from build123d import *

# Parameters (mm, degrees)
AUFSATZ_LINEAR_AUSTRAGEN1_DEPTH = 18
F_8_0_8_DURCHMESSER_BOHRUNG1_D  = 8


with BuildPart() as part:
    # Skizze1 → Aufsatz-Linear austragen1 (new body)
    with BuildSketch(Plane(origin=(0, 0, 0), x_dir=(1, 0, 0), z_dir=(0, 1, 0))):
        with BuildLine():
            Line((2.016149839, 16.814436139), (2.801632478, 16.701526227))
            ThreePointArc((2.801632478, 16.701526227), (3.101511816, 16.50942794), (3.153726656, 16.157145411))
            ThreePointArc((3.153726656, 16.157145411), (3.283097912, 15.001210678), (4.189865695, 14.272723054))
            ThreePointArc((4.189865695, 14.272723054), (5.346528394, 14.395402891), (6.080251078, 15.297938189))
            ThreePointArc((6.080251078, 15.297938189), (6.314618428, 15.566081904), (6.67074882, 15.565580692))
            Line((6.67074882, 15.565580692), (7.392603495, 15.235948392))
            ThreePointArc((7.392603495, 15.235948392), (7.626215271, 14.967145662), (7.577065585, 14.614422431))
            ThreePointArc((7.577065585, 14.614422431), (7.375531949, 13.468863082), (8.040330584, 12.514418319))
            ThreePointArc((8.040330584, 12.514418319), (9.184703221, 12.306259221), (10.142978558, 12.965521931))
            ThreePointArc((10.142978558, 12.965521931), (10.443397198, 13.156775028), (10.784960599, 13.055960593))
            Line((10.784960599, 13.055960593), (11.384706937, 12.536310754))
            ThreePointArc((11.384706937, 12.536310754), (11.533125314, 12.212580381), (11.386592918, 11.887991985))
            ThreePointArc((11.386592918, 11.887991985), (10.870481446, 10.845614425), (11.239452902, 9.742535963))
            ThreePointArc((11.239452902, 9.742535963), (12.278825211, 9.220401742), (13.384019433, 9.582982318))
            ThreePointArc((13.384019433, 9.582982318), (13.726151231, 9.68185061), (14.025476205, 9.488890337))
            Line((14.025476205, 9.488890337), (14.454526325, 8.821321899))
            ThreePointArc((14.454526325, 8.821321899), (14.505727329, 8.468890591), (14.273683407, 8.198733253))
            ThreePointArc((14.273683407, 8.198733253), (13.48480638, 7.343984713), (13.528058784, 6.181637408))
            ThreePointArc((13.528058784, 6.181637408), (14.378227002, 5.387828273), (15.540803845, 5.424352595))
            ThreePointArc((15.540803845, 5.424352595), (15.896931319, 5.422826359), (16.129768337, 5.153352743))
            Line((16.129768337, 5.153352743), (16.353363149, 4.39194813))
            ThreePointArc((16.353363149, 4.39194813), (16.30319878, 4.039367777), (16.004442149, 3.845528037))
            ThreePointArc((16.004442149, 3.845528037), (15.006709693, 3.247655161), (14.720738993, 2.120205477))
            ThreePointArc((14.720738993, 2.120205477), (15.312827547, 1.119031124), (16.43860195, 0.826540208))
            ThreePointArc((16.43860195, 0.826540208), (16.779873768, 0.724743092), (16.92735976, 0.400587283))
            Line((16.92735976, 0.400587283), (16.927384943, -0.392969032))
            ThreePointArc((16.927384943, -0.392969032), (16.779919219, -0.717134467), (16.438653365, -0.818952866))
            ThreePointArc((16.438653365, -0.818952866), (15.31289583, -1.111513974), (14.72086967, -2.112726767))
            ThreePointArc((14.72086967, -2.112726767), (15.006911068, -3.240157147), (16.004679484, -3.837967426))
            ThreePointArc((16.004679484, -3.837967426), (16.303447834, -4.031788426), (16.353634362, -4.384365253))
            Line((16.353634362, -4.384365253), (16.130087875, -5.145784056))
            ThreePointArc((16.130087875, -5.145784056), (15.897267592, -5.415272618), (15.541139845, -5.416820955))
            ThreePointArc((15.541139845, -5.416820955), (14.378559411, -5.380368734), (13.528440231, -6.17423233))
            ThreePointArc((13.528440231, -6.17423233), (13.485261098, -7.336581031), (14.274190264, -8.191279641))
            ThreePointArc((14.274190264, -8.191279641), (14.50625071, -8.4614223), (14.455071961, -8.813856467))
            Line((14.455071961, -8.813856467), (14.026064211, -9.481452135))
            ThreePointArc((14.026064211, -9.481452135), (13.726751084, -9.674431463), (13.384612796, -9.5755843))
            ThreePointArc((13.384612796, -9.5755843), (12.279394816, -9.213071892), (11.240054215, -9.735272184))
            ThreePointArc((11.240054215, -9.735272184), (10.871152669, -10.838372629), (11.387328235, -11.880716971))
            ThreePointArc((11.387328235, -11.880716971), (11.533880622, -12.205295936), (11.385482792, -12.529035323))
            Line((11.385482792, -12.529035323), (10.785769436, -13.048723226))
            ThreePointArc((10.785769436, -13.048723226), (10.444212034, -13.149559283), (10.143781215, -12.95832463))
            ThreePointArc((10.143781215, -12.95832463), (9.185463876, -12.299120634), (8.041103048, -12.50735206))
            ThreePointArc((8.041103048, -12.50735206), (7.376365299, -13.461837611), (7.577969791, -14.607383145))
            ThreePointArc((7.577969791, -14.607383145), (7.627141314, -14.96010296), (7.393546714, -15.228920127))
            Line((7.393546714, -15.228920127), (6.671712961, -15.558598241))
            ThreePointArc((6.671712961, -15.558598241), (6.315582234, -15.559121889), (6.081198001, -15.29099244))
            ThreePointArc((6.081198001, -15.29099244), (5.347418475, -14.388501644), (4.19074673, -14.265894532))
            ThreePointArc((4.19074673, -14.265894532), (3.284025875, -14.994438446), (3.154726497, -16.150379885))
            ThreePointArc((3.154726497, -16.150379885), (3.102533573, -16.502665289), (2.802666647, -16.694782268))
            Line((2.802666647, -16.694782268), (2.017191175, -16.807742033))
            ThreePointArc((2.017191175, -16.807742033), (1.675338716, -16.707910849), (1.525989487, -16.384608858))
            ThreePointArc((1.525989487, -16.384608858), (1.076194227, -15.311945698), (0.00091823, -14.868432948))
            ThreePointArc((0.00091823, -14.868432948), (-1.074328599, -15.312012929), (-1.524056781, -16.384702774))
            ThreePointArc((-1.524056781, -16.384702774), (-1.673385793, -16.708013697), (-2.015231609, -16.807866313))
            Line((-2.015231609, -16.807866313), (-2.800714248, -16.6949564))
            ThreePointArc((-2.800714248, -16.6949564), (-3.100593586, -16.502858113), (-3.152808426, -16.150575585))
            ThreePointArc((-3.152808426, -16.150575585), (-3.282179682, -14.994640851), (-4.188947465, -14.266153228))
            ThreePointArc((-4.188947465, -14.266153228), (-5.345610164, -14.388833064), (-6.079332848, -15.291368363))
            ThreePointArc((-6.079332848, -15.291368363), (-6.313700199, -15.559512077), (-6.66983059, -15.559010865))
            Line((-6.66983059, -15.559010865), (-7.391685265, -15.229378565))
            ThreePointArc((-7.391685265, -15.229378565), (-7.625297041, -14.960575836), (-7.576147355, -14.607852605))
            ThreePointArc((-7.576147355, -14.607852605), (-7.374613719, -13.462293255), (-8.039412354, -12.507848493))
            ThreePointArc((-8.039412354, -12.507848493), (-9.183784991, -12.299689395), (-10.142060328, -12.958952104))
            ThreePointArc((-10.142060328, -12.958952104), (-10.442478968, -13.150205201), (-10.784042369, -13.049390766))
            Line((-10.784042369, -13.049390766), (-11.383788707, -12.529740927))
            ThreePointArc((-11.383788707, -12.529740927), (-11.532207084, -12.206010554), (-11.385674688, -11.881422159))
            ThreePointArc((-11.385674688, -11.881422159), (-10.869563216, -10.839044599), (-11.238534672, -9.735966136))
            ThreePointArc((-11.238534672, -9.735966136), (-12.277906981, -9.213831915), (-13.383101203, -9.576412492))
            ThreePointArc((-13.383101203, -9.576412492), (-13.725233001, -9.675280783), (-14.024557975, -9.482320511))
            Line((-14.024557975, -9.482320511), (-14.453608095, -8.814752072))
            ThreePointArc((-14.453608095, -8.814752072), (-14.5048091, -8.462320765), (-14.272765177, -8.192163427))
            ThreePointArc((-14.272765177, -8.192163427), (-13.48388815, -7.337414887), (-13.527140554, -6.175067581))
            ThreePointArc((-13.527140554, -6.175067581), (-14.377308772, -5.381258446), (-15.539885615, -5.417782768))
            ThreePointArc((-15.539885615, -5.417782768), (-15.896013089, -5.416256533), (-16.128850107, -5.146782917))
            Line((-16.128850107, -5.146782917), (-16.352444919, -4.385378304))
            ThreePointArc((-16.352444919, -4.385378304), (-16.30228055, -4.03279795), (-16.003523919, -3.838958211))
            ThreePointArc((-16.003523919, -3.838958211), (-15.005791463, -3.241085334), (-14.719820763, -2.113635651))
            ThreePointArc((-14.719820763, -2.113635651), (-15.311909317, -1.112461298), (-16.43768372, -0.819970382))
            ThreePointArc((-16.43768372, -0.819970382), (-16.778955538, -0.718173266), (-16.926441531, -0.394017456))
            Line((-16.926441531, -0.394017456), (-16.926466713, 0.399538858))
            ThreePointArc((-16.926466713, 0.399538858), (-16.779000989, 0.723704294), (-16.437735135, 0.825522693))
            ThreePointArc((-16.437735135, 0.825522693), (-15.3119776, 1.118083801), (-14.71995144, 2.119296594))
            ThreePointArc((-14.71995144, 2.119296594), (-15.005992838, 3.246726973), (-16.003761254, 3.844537253))
            ThreePointArc((-16.003761254, 3.844537253), (-16.302529604, 4.038358252), (-16.352716132, 4.39093508))
            Line((-16.352716132, 4.39093508), (-16.129169645, 5.152353882))
            ThreePointArc((-16.129169645, 5.152353882), (-15.896349362, 5.421842445), (-15.540221615, 5.423390781))
            ThreePointArc((-15.540221615, 5.423390781), (-14.377641181, 5.38693856), (-13.527522001, 6.180802156))
            ThreePointArc((-13.527522001, 6.180802156), (-13.484342868, 7.343150858), (-14.273272034, 8.197849468))
            ThreePointArc((-14.273272034, 8.197849468), (-14.505332481, 8.467992126), (-14.454153731, 8.820426293))
            Line((-14.454153731, 8.820426293), (-14.025145981, 9.488021961))
            ThreePointArc((-14.025145981, 9.488021961), (-13.725832854, 9.68100129), (-13.383694566, 9.582154127))
            ThreePointArc((-13.383694566, 9.582154127), (-12.278476586, 9.219641719), (-11.239135985, 9.741842011))
            ThreePointArc((-11.239135985, 9.741842011), (-10.870234439, 10.844942456), (-11.386410005, 11.887286797))
            ThreePointArc((-11.386410005, 11.887286797), (-11.532962392, 12.211865763), (-11.384564562, 12.53560515))
            Line((-11.384564562, 12.53560515), (-10.784851206, 13.055293052))
            ThreePointArc((-10.784851206, 13.055293052), (-10.443293804, 13.156129109), (-10.142862985, 12.964894457))
            ThreePointArc((-10.142862985, 12.964894457), (-9.184545646, 12.305690461), (-8.040184818, 12.513921887))
            ThreePointArc((-8.040184818, 12.513921887), (-7.375447069, 13.468407437), (-7.577051561, 14.613952971))
            ThreePointArc((-7.577051561, 14.613952971), (-7.626223084, 14.966672786), (-7.392628484, 15.235489954))
            Line((-7.392628484, 15.235489954), (-6.670794731, 15.565168067))
            ThreePointArc((-6.670794731, 15.565168067), (-6.314664004, 15.565691715), (-6.080279771, 15.297562267))
            ThreePointArc((-6.080279771, 15.297562267), (-5.346500245, 14.395071471), (-4.1898285, 14.272464359))
            ThreePointArc((-4.1898285, 14.272464359), (-3.283107646, 15.001008272), (-3.153808267, 16.156949712))
            ThreePointArc((-3.153808267, 16.156949712), (-3.101615343, 16.509235115), (-2.801748417, 16.701352094))
            Line((-2.801748417, 16.701352094), (-2.016272945, 16.814311859))
            ThreePointArc((-2.016272945, 16.814311859), (-1.674420486, 16.714480675), (-1.525071257, 16.391178685))
            ThreePointArc((-1.525071257, 16.391178685), (-1.075275997, 15.318515525), (0, 14.875002774))
            ThreePointArc((0, 14.875002774), (1.075246829, 15.318582755), (1.524975011, 16.3912726))
            ThreePointArc((1.524975011, 16.3912726), (1.674304023, 16.714583523), (2.016149839, 16.814436139))
        make_face()
    extrude(amount=AUFSATZ_LINEAR_AUSTRAGEN1_DEPTH)

    # Ø8.0 (8) Durchmesser Bohrung1 (through all)
    with Locations(Plane(origin=(0, 18, 0), x_dir=(1, 0, 0), z_dir=(0, 1, 0))):
        with Locations((0, 0)):
            Hole(F_8_0_8_DURCHMESSER_BOHRUNG1_D / 2)


solid = part.part
Part model, mm, in its own coordinate system. Coordinates: 2 decimals unless noted, no trailing zeros. Loops run counter-clockwise (first coordinate to the right, second up) from the corner with the lowest first, then second, coordinate; pieces in that order, holes last. Notation, with made-up numbers: (-34.75, 1.25) - (-15.75, 1.25) arc R26 cw to (-15.75, 30.25) - close; hole circle Ø6 at (13.25, -30). An arc over 180 degrees is marked (long way). Write each question's results on one line, items separated by ' | '. Start each with the question number.
Q1. Drop flat-ended pins along their axis: pin 1 Ø8 at (x, y) = (-8, 5) entering from +Z; pin 2 Ø4 at (y, z) = (3, -6) entering from -X; pin 3 Ø3 at (x, y) = (11.5, 3.5) entering from +Z. Give the stop position or say it passes through.
Q2. Slice it at B-B on x = 9. Give the cut face in (y, z).
Q3. Two-plate mould, pull along Z, no slides. Class faces 1 (the flat face through (-4, 18, 3)), 2 (the cylindrical face through (0.867, 8.874, 3.905)): +Z half, -Z half, draft (parallel to the pull), parting line (faces both ways), or undercut.
Q4. Slice it at A-A on z = -10.5. Give the cut face in (x, y), and give its area (3 significant figures).
Q5. Probe line 1 along Z through (x, y) = (0, 5) (3 decimals); line 2 along X through (y, z) = (4.75, -2); line 3 along Z through (x, y) = (-6.5, 1.25). List the from-to ranges inside material, lowest first.
Answer:
1) pin 1: stops at z = 15.6 | pin 2: stops at x = -16.37 | pin 3: stops at z = 13.15
2) outline: (0, -12.28) - (18, -12.28) - (18, 12.27) - (0, 12.27) - close
3) face 1: draft | face 2: undercut
4) outline: (-10.89, 0) - (10.89, 0) - (10.89, 18) - (-10.89, 18) - close | area: 392 mm2
5) line 1: z = -14.875 to -4, 4 to 14.868 | line 2: x = -14.74 to -3.46, 3.46 to 14.74 | line 3: z = -15.6 to 15.6
